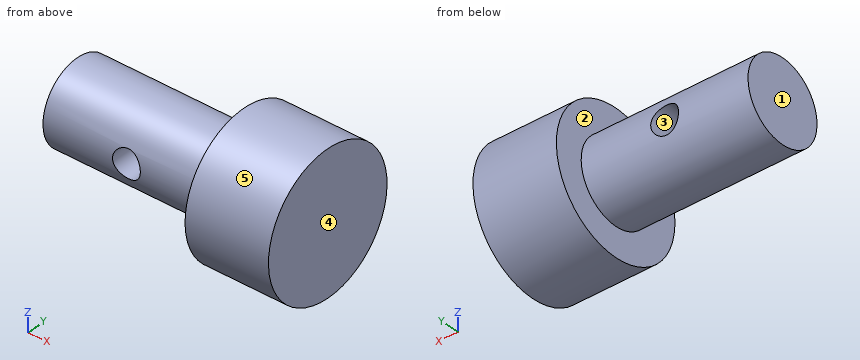
```python
from build123d import *

# Parameters (mm, degrees)
SKETCH2_R               = 1.455
BOSS_EXTRUDE3_DEPTH     = 6
SKETCH3_R               = 2.5
BOSS_EXTRUDE4_DEPTH     = 3
CUT_EXTRUDE1_DEPTH      = 10.669539803
CUT_EXTRUDE1_DEPTH_BACK = 10.669539803
SKETCH4_R               = 0.5


with BuildPart() as part:
    # Sketch2 → Boss-Extrude3 (new body)
    with BuildSketch(Plane(origin=(0, 0, 0), x_dir=(0, 0, -1), z_dir=(1, 0, 0))):
        Circle(SKETCH2_R)
    extrude(amount=BOSS_EXTRUDE3_DEPTH)

    # Sketch3 → Boss-Extrude4 (add)
    with BuildSketch(Plane(origin=(6, 0, 0), x_dir=(0, 0, -1), z_dir=(1, 0, 0))):
        Circle(SKETCH3_R)
    extrude(amount=BOSS_EXTRUDE4_DEPTH)

    # Sketch4 → Cut-Extrude1 (cut, two sides: drawn at the far end of the back side and taken through both)
    with BuildSketch(Plane(origin=(0, 0, 0), x_dir=(1, 0, 0), z_dir=(0, 1, 0)).offset(-CUT_EXTRUDE1_DEPTH_BACK)):
        with Locations(Location((3, 0, 0), (0, 0, 270))):
            Circle(SKETCH4_R)
    extrude(amount=CUT_EXTRUDE1_DEPTH + CUT_EXTRUDE1_DEPTH_BACK, mode=Mode.SUBTRACT)


solid = part.part
```
Verification items for the finished model (mm, model axes). Face numbers are marked on the shaded views. A direction names the side the tool comes from. Round coordinates to 2 decimals unless told otherwise and drop trailing zeros. Order: outer loops, then holes, each group sorted by start corner. A loop starts at its lowest first (then second) coordinate and runs counter-clockwise, first axis right, second up.
1) Material ranges on line 1 (X direction, y = -0.5, z = 0); line 2 (Z direction, x = 3, y = 0.45); line 3 (X direction, y = -0.8, z = -1.6), recorded low to high.
Geometry says:
line 1: x = 0 to 2.5, 3.5 to 9
line 2: z = -1.38 to -0.5, 0.5 to 1.38
line 3: x = 6 to 9
2) Cross-section at D-D, the plane z = 0.65. Record the cut outline in (x, y), plus the area to 3 significant figures.
Geometry says:
outline: (0, -1.3) - (6, -1.3) - (6, -2.41) - (9, -2.41) - (9, 2.41) - (6, 2.41) - (6, 1.3) - (0, 1.3) - close
area: 30.1 mm2
3) Cross-section at B-B, the plane y = 0. Record the cut outline in (x, z) (3 decimals).
Geometry says:
outline: (0, -1.455) - (6, -1.455) - (6, -2.5) - (9, -2.5) - (9, 2.5) - (6, 2.5) - (6, 1.455) - (0, 1.455) - close; hole circle Ø1 at (3, 0)
4) Tool access check on the marked faces 1 and 2. Record the directions out of +Z, -Z, +X, -X, +Y, -Y that give a thin tool (end or side, any length) a straight path to the whole face; none if there is none.
Geometry says:
face 1: +Z, -Z, -X, +Y, -Y
face 2: -X
5) Draft check along Z on the marked faces 3, 4 and 5. Enter one of: +Z half, -Z half, draft (parallel to the pull), parting line (faces both ways), or undercut.
Geometry says:
face 3: undercut
face 4: draft
face 5: parting line
6) Cross-section at A-A, the plane z = 0. Record the cut outline in (x, y) (3 decimals).
Geometry says:
outline: (0, -1.455) - (2.5, -1.455) - (2.5, 1.455) - (0, 1.455) - close; (3.5, -1.455) - (6, -1.455) - (6, -2.5) - (9, -2.5) - (9, 2.5) - (6, 2.5) - (6, 1.455) - (3.5, 1.455) - close
7) Cross-section at C-C, the plane x = 6.25. Record the cut outline in (y, z).
Geometry says:
outline: circle Ø5 at (0, 0)
8) Depth check by flat-ended pin: pin 1 (3 mm diameter, centred on x = 2, y = -0.5, fed in from +Z) (3 decimals). Enter the tip coordinate at first touch or a pass-through.
Geometry says:
pin 1: stops at z = 1.455
